Source: CAD feature listing. Evaluate the final solid. Frame: model axes, mm. Face numbers are marked on the shaded views. A direction names the side the tool comes from. Coordinates: 2 decimals unless noted, no trailing zeros. Loops run counter-clockwise (first coordinate to the right, second up) from the corner with the lowest first, then second, coordinate; pieces in that order, holes last.
Item 1: Section query C-C, the plane y = 16. Return the cut outline in (x, z), then the cut area to 3 significant figures.
Item 2: Reachability of the marked faces 5, 6, 7 and 8 from +Z, -Z, +X, -X, +Y, -Y: full face, straight path, thin tool, end or side. Return the list, or none.
Item 3: Pin query (flat end, axial travel): pin 1 Ø2.5 at (x, z) = (20, -38) entering from +Y; pin 2 Ø20 at (x, y) = (4, -18.5) entering from -Z; pin 3 Ø4 at (y, z) = (50, -38.5) entering from +X. Return the tip coordinate at first contact, or that it passes through.
Item 4: Section query D-D, the plane x = 18. Return the cut outline in (y, z).
Item 5: Line query: probe 1 along X at (y, z) = (-26.6, 0); probe 2 along Y at (x, z) = (7, 1); probe 3 along Y at (x, z) = (-8, -4.5). Output: solid intervals per line, ascending.
Item 6: Section query B-B, the plane z = 0. Return the cut outline in (x, y), then the cut area to 3 significant figures.
Item 7: Section query A-A, the plane x = 25. Return the cut outline in (y, z).
Item 8: Pull-direction query (Z, two-part tool) for the marked faces 1, 2, 3 and 4; classes: +Z half, -Z half, draft (parallel to the pull), parting line (faces both ways), or undercut.
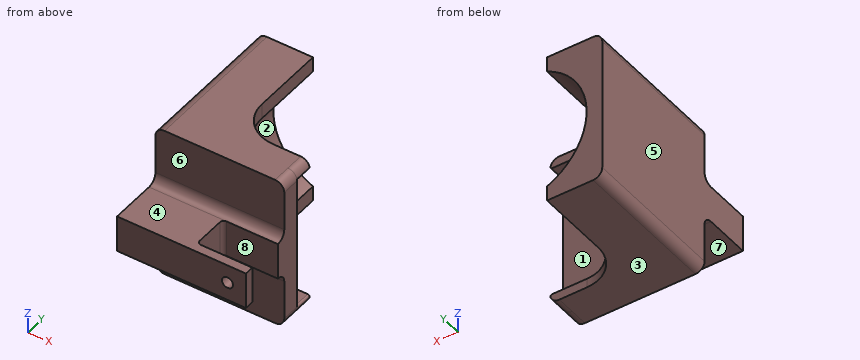
```python
from build123d import *

# Parameters (mm, degrees)
EXTRUDE_1_DEPTH     = 10
EXTRUDE_2_DEPTH     = 70
SKETCH_6_W          = 70
SKETCH_6_H          = 20
EXTRUDE_3_DEPTH     = 30
SKETCH_8_R          = 3
CUT_EXTRUDE_5_DEPTH = 15
FILLET_2_R          = 5
SKETCH_9_W          = 20
SKETCH_9_H          = 20
CUT_EXTRUDE_6_DEPTH = 30
FILLET_4_R          = 2
CUT_EXTRUDE_7_DEPTH = 121.474063599


with BuildPart() as part:
    # 草圖2 → 填料-伸長1 (new body)
    with BuildSketch(Plane(origin=(0, 0, 0), x_dir=(1, 0, 0), z_dir=(0, 1, 0))):
        with BuildLine():
            Line((-30, 41.5), (30, 41.5))
            ThreePointArc((30, 41.5), (33.535533906, 40.035533906), (35, 36.5))
            Line((35, 36.5), (35, -36.5))
            ThreePointArc((35, -36.5), (33.535533906, -40.035533906), (30, -41.5))
            Line((30, -41.5), (-30, -41.5))
            ThreePointArc((-30, -41.5), (-33.535533906, -40.035533906), (-35, -36.5))
            Line((-35, -36.5), (-35, 36.5))
            ThreePointArc((-35, 36.5), (-33.535533906, 40.035533906), (-30, 41.5))
        make_face()
    extrude(amount=EXTRUDE_1_DEPTH)

    # 草圖3 → 填料-伸長2 (add)
    with BuildSketch(Plane(origin=(0, 10, 0), x_dir=(1, 0, 0), z_dir=(0, 1, 0))):
        with BuildLine():
            Line((-35, 36.5), (-35, -36.5))
            ThreePointArc((-35, -36.5), (-33.535533906, -40.035533906), (-30, -41.5))
            Line((-30, -41.5), (30, -41.5))
            ThreePointArc((30, -41.5), (33.061862178, -40.452847075), (34.841229183, -37.75))
            ThreePointArc((34.841229183, -37.75), (34.663552761, -36.887627564), (33.872983346, -36.5))
            Line((33.872983346, -36.5), (10, -36.5))
            ThreePointArc((10, -36.5), (-26.5, 0), (10, 36.5))
            Line((10, 36.5), (33.872983346, 36.5))
            ThreePointArc((33.872983346, 36.5), (34.663552761, 36.887627564), (34.841229183, 37.75))
            ThreePointArc((34.841229183, 37.75), (33.061862178, 40.452847075), (30, 41.5))
            Line((30, 41.5), (-30, 41.5))
            ThreePointArc((-30, 41.5), (-33.535533906, 40.035533906), (-35, 36.5))
        make_face()
    extrude(amount=EXTRUDE_2_DEPTH)

    # 草圖6 → 填料-伸長3 (add)
    with BuildSketch(Plane.XZ):
        Rectangle(SKETCH_6_W, SKETCH_6_H)
    extrude(amount=EXTRUDE_3_DEPTH)

    # 草圖8 → 除料-伸長5 (cut)
    with BuildSketch(Plane.XZ.offset(30)):
        with Locations(Location((25, 0, 0), (0, 0, 270))):
            Circle(SKETCH_8_R)
    extrude(amount=-CUT_EXTRUDE_5_DEPTH, mode=Mode.SUBTRACT)

    # 圓角2
    fillet_2_edges = [part.edges().sort_by_distance(p)[0] for p in [
        (0, 0, -10),
        (0, 0, 10),
    ]]
    fillet(fillet_2_edges, radius=FILLET_2_R)

    # 草圖9 → 除料-伸長6 (cut)
    with BuildSketch(Plane(origin=(35, 0, 0), x_dir=(0, 0, -1), z_dir=(1, 0, 0))):
        with Locations((0, -15)):
            Rectangle(SKETCH_9_W, SKETCH_9_H)
    extrude(amount=-CUT_EXTRUDE_6_DEPTH, mode=Mode.SUBTRACT)

    # 圓角4
    fillet_4_edges = [part.edges().sort_by_distance(p)[0] for p in [
        (5, -25, 0),
        (5, -5, 0),
    ]]
    fillet(fillet_4_edges, radius=FILLET_4_R)

    # 草圖10 → 除料-伸長7 (cut, through all)
    with BuildSketch(Plane.XY.offset(41.5)):
        with BuildLine():
            Line((35, 80), (-5, 80))
            Line((-5, 80), (-5, 40))
            ThreePointArc((-5, 40), (0.857864376, 25.857864376), (15, 20))
            Line((15, 20), (35, 20))
            Line((35, 20), (35, 80))
        make_face()
    extrude(amount=-CUT_EXTRUDE_7_DEPTH, mode=Mode.SUBTRACT)


solid = part.part
```
Verdict:
1. outline: (-35, -36.5) arc R5 ccw to (-30, -41.5) - (30, -41.5) arc R5 ccw to (34.84, -37.75) arc R1 ccw to (33.87, -36.5) - (10, -36.5) arc R36.5 cw to (10, 36.5) - (33.87, 36.5) arc R1 ccw to (34.84, 37.75) arc R5 ccw to (30, 41.5) - (-30, 41.5) arc R5 ccw to (-35, 36.5) - close
1. area: 1,870 mm2
2. face 5: +Z, -Z, -X, +Y, -Y
2. face 6: +Z, +X, -X, -Y
2. face 7: -Z, +X, -X, -Y
2. face 8: +Z, -Z, +X
3. pin 1: stops at y = 20
3. pin 2: stops at z = -10
3. pin 3: stops at x = -5
4. outline: (-30, -10) - (-25, -10) - (-25, 10) - (-30, 10) - close; (-5, -10) arc R5 cw to (0, -15) - (0, -41.5) - (20, -41.5) - (20, -36.5) - (10, -36.5) - (10, 36.5) - (20, 36.5) - (20, 41.5) - (0, 41.5) - (0, 15) arc R5 cw to (-5, 10) - close
5. probe 1: x = -35 to 22, 28 to 35
5. probe 2: y = -30 to -25, -5 to 10
5. probe 3: y = -30 to 10
6. outline: (-35, -30) - (22, -30) - (22, -25) - (7, -25) arc R2 cw to (5, -23) - (5, -7) arc R2 cw to (7, -5) - (35, -5) - (35, 10) - (-26.5, 10) - (-26.5, 80) - (-35, 80) - close; (28, -30) - (35, -30) - (35, -25) - (28, -25) - close
6. area: 2,770 mm2
7. outline: (-30, -10) - (-25, -10) - (-25, -3) - (-30, -3) - close; (-30, 3) - (-25, 3) - (-25, 10) - (-30, 10) - close; (-5, -10) arc R5 cw to (0, -15) - (0, -41.5) - (20, -41.5) - (20, -36.5) - (10, -36.5) - (10, 36.5) - (20, 36.5) - (20, 41.5) - (0, 41.5) - (0, 15) arc R5 cw to (-5, 10) - close
8. face 1: undercut
8. face 2: undercut
8. face 3: -Z half
8. face 4: +Z half
